Input: part model. Units: mm. Frame: model coordinates. A direction names the side the tool comes from. Give positions to 0.01 mm unless a question says otherwise; leave off trailing zeros. Loops run counter-clockwise (first coordinate to the right, second up) from the corner with the lowest first, then second, coordinate; pieces in that order, holes last. Notation, with made-up numbers: (-36, 79) -> (1, 79) arc R30 cw to (1, 102) -> close; hole circle Ø10 at (-32, -28). An arc over 180 degrees is marked (long way). Answer as a JSON object with one key per item and string values.
```python
from build123d import *

# Parameters (mm, degrees)
Y_KSEKLIK_EKSTR_ZYON1_DEPTH = 15
BOSS_EXTRUDE1_DEPTH         = 10


with BuildPart() as part:
    # Çizim1 → Yükseklik-Ekstrüzyon1 (new body)
    with BuildSketch(Plane.XY):
        with BuildLine():
            Line((-90.996604912, -49.609404393), (-40.996604912, -80.724218798))
            ThreePointArc((-40.996604912, -80.724218798), (-0.437932375, -81.729892604), (20.137283846, -46.763082981))
            Line((20.137283846, -46.763082981), (20.137283846, 15.466545829))
            ThreePointArc((20.137283846, 15.466545829), (-0.437932375, 50.433355451), (-40.996604912, 49.427681645))
            Line((-40.996604912, 49.427681645), (-90.996604912, 18.31286724))
            ThreePointArc((-90.996604912, 18.31286724), (-109.862716154, -15.648268576), (-90.996604912, -49.609404393))
        make_face()
        with BuildLine():
            Line((-83.071396628, -36.873978462), (-33.071396628, -67.988792867))
            ThreePointArc((-33.071396628, -67.988792867), (-7.722226292, -68.617338995), (5.137283846, -46.763082981))
            Line((5.137283846, -46.763082981), (5.137283846, 15.466545829))
            ThreePointArc((5.137283846, 15.466545829), (-7.722226292, 37.320801843), (-33.071396628, 36.692255714))
            Line((-33.071396628, 36.692255714), (-83.071396628, 5.577441309))
            ThreePointArc((-83.071396628, 5.577441309), (-94.862716154, -15.648268576), (-83.071396628, -36.873978462))
        make_face(mode=Mode.SUBTRACT)
    extrude(amount=Y_KSEKLIK_EKSTR_ZYON1_DEPTH)

    # Çizim1<3> → Boss-Extrude1 (add)
    with BuildSketch(Plane.XY):
        with BuildLine():
            Line((-83.071396628, -36.873978462), (-33.071396628, -67.988792867))
            ThreePointArc((-33.071396628, -67.988792867), (-7.722226292, -68.617338995), (5.137283846, -46.763082981))
            Line((5.137283846, -46.763082981), (5.137283846, 15.466545829))
            ThreePointArc((5.137283846, 15.466545829), (-7.722226292, 37.320801843), (-33.071396628, 36.692255714))
            Line((-33.071396628, 36.692255714), (-83.071396628, 5.577441309))
            ThreePointArc((-83.071396628, 5.577441309), (-94.862716154, -15.648268576), (-83.071396628, -36.873978462))
        make_face()
    extrude(amount=BOSS_EXTRUDE1_DEPTH)


solid = part.part
```
Q1. Pin query (flat end, axial travel): pin 1 (5 mm diameter, centred on x = -30, z = 9.5, fed in from +Y); pin 2 (5 mm diameter, centred on x = -55.5, z = 9.5, fed in from +Y); pin 3 (1.5 mm diameter, centred on y = -26.5, z = 11.5, fed in from -X). Return the tip coordinate at first contact, or that it passes through.
Evaluation:
{"pin 1": "stops at y = 54.73", "pin 2": "stops at y = 41.96", "pin 3": "stops at x = -108.57"}
Q2. Draft query along X for faces 3 (the flat face through (-60, -52, 15)), 4 (the flat face through (-58.421, -52.214, 12.465)), 5 (the cylindrical face through (-109.86, -15.08, 7.4)), 6 (the cylindrical face through (0.08, 50.14, 7.4)). Return one class per face: +X half, -X half, draft (parallel to the pull), parting line (faces both ways), or undercut.
Evaluation:
{"face 3": "draft", "face 4": "undercut", "face 5": "-X half", "face 6": "parting line"}
Q3. Section D-D, the plane y = 44. Return the cut outline in (x, z), then the cut area to 3 significant figures.
Evaluation:
{"outline": "(-49.72, 0) -> (8.17, 0) -> (8.17, 15) -> (-49.72, 15) -> close", "area": "868 mm2"}
Q4. Section A-A, the plane z = 12.75. Return the cut outline in (x, y).
Evaluation:
{"outline": "(-91, -49.61) -> (-41, -80.72) arc R40 ccw to (20.14, -46.76) -> (20.14, 15.47) arc R40 ccw to (-41, 49.43) -> (-91, 18.31) arc R40 ccw to start; hole (-83.07, -36.87) -> (-33.07, -67.99) arc R25 ccw to (5.14, -46.76) -> (5.14, 15.47) arc R25 ccw to (-33.07, 36.69) -> (-83.07, 5.58) arc R25 ccw to start"}
Q5. Access query for faces 1 (the flat face through (-57.721, 21.353, 12.465)), 2 (the flat face through (-65.647, 34.088, 7.395)). Directions: +Z, -Z, +X, -X, +Y, -Y. A direction counts if a zero-diameter tool reaches every point of the face in a straight line with its end or side. Return the directions, or none.
Evaluation:
{"face 1": "+Z", "face 2": "+Z, -Z, -X, +Y"}
Q6. Ray query, line 1 along Z through (x, y) = (-8.5, -66.5); line 2 along Y through (x, z) = (-61.5, 13.25); line 3 along Y through (x, z) = (-57.5, 11.75). Return the intervals inside material, ascending.
Evaluation:
{"line 1": "z = 0 to 10", "line 2": "y = -67.97 to -50.3, 19 to 36.67", "line 3": "y = -70.45 to -52.79, 21.49 to 39.16"}
Q7. Section C-C, the plane x = -55.5. Return the cut outline in (y, z), then the cut area to 3 significant figures.
Evaluation:
{"outline": "(-71.7, 0) -> (40.4, 0) -> (40.4, 15) -> (22.74, 15) -> (22.74, 10) -> (-54.03, 10) -> (-54.03, 15) -> (-71.7, 15) -> close", "area": "1,300 mm2"}
Q8. Section B-B, the plane y = 27. Return the cut outline in (x, z).
Evaluation:
{"outline": "(-77.04, 0) -> (18.44, 0) -> (18.44, 15) -> (2.32, 15) -> (2.32, 10) -> (-48.65, 10) -> (-48.65, 15) -> (-77.04, 15) -> close"}
